Here's how the part is built. I have some questions about the finished solid (model axes, mm). A direction names the side the tool comes from. Coordinates: 2 decimals unless noted, no trailing zeros. Write each loop counter-clockwise with the first axis right and the second up, starting at its lowest first coordinate (ties: lowest second). Pieces come first, ordered by that corner, then holes. Notation, with made-up numbers: (-34.75, 52) -> (-27.75, 52) arc R12 ccw to (-27.75, 68) -> close; hole circle Ø9 at (5.5, 1). An arc over 180 degrees is marked (long way). Put each result on its own line as item: value.
```python
from build123d import *

# Parameters (mm, degrees)
SKETCH_1_W               = 42
SKETCH_1_H               = 42
EXTRUDE_1_DEPTH          = 65
SKETCH_2_R               = 18
EXTRUDE_2_DEPTH          = 22
EXTRUDE_3_DEPTH          = 19
SKETCH_4_R               = 11
EXTRUDE_4_DEPTH          = 2
SKETCH_6_W               = 43
SKETCH_6_H               = 1
CUT_EXTRUDE_1_DEPTH      = 2
PATTERN_CIRCULAR_1_COUNT = 4
HOLE_WIZARD_M3_1_D       = 2.5
HOLE_WIZARD_M3_1_DEPTH   = 7.5
HOLE_WIZARD_M3_1_TIP     = 0.751075774
SKETCH_9_W               = 16
SKETCH_9_H               = 9.5
EXTRUDE_5_DEPTH          = 8


with BuildPart() as part:
    # 草图1 → 凸台-拉伸1 (new body)
    with BuildSketch(Plane.XY):
        Rectangle(SKETCH_1_W, SKETCH_1_H)
    extrude(amount=EXTRUDE_1_DEPTH)

    # 草图2 → 凸台-拉伸2 (add)
    with BuildSketch(Plane.XY.offset(65)):
        Circle(SKETCH_2_R)
    extrude(amount=EXTRUDE_2_DEPTH)

    # 草图3 → 凸台-拉伸3 (add)
    with BuildSketch(Plane.XY.offset(87)):
        with BuildLine():
            Line((-2.645751311, 3), (2.645751311, 3))
            ThreePointArc((2.645751311, 3), (0, -4), (-2.645751311, 3))
        make_face()
    extrude(amount=EXTRUDE_3_DEPTH)

    # 草图4 → 凸台-拉伸4 (add)
    with BuildSketch(Plane.XY.offset(87)):
        Circle(SKETCH_4_R)
    extrude(amount=EXTRUDE_4_DEPTH)

    # 草图6 → 切除-拉伸1 (cut)
    with BuildSketch(Plane(origin=(0, 21, 0), x_dir=(1, 0, 0), z_dir=(0, 1, 0))):
        with Locations((0, -60)):
            Rectangle(SKETCH_6_W, SKETCH_6_H)
    cut_extrude_1 = extrude(amount=-CUT_EXTRUDE_1_DEPTH, mode=Mode.SUBTRACT)

    # 阵列(圆周)1: 切除-拉伸1 ×4 about axis
    pattern_circular_1_axis = Axis((0, 0, 0), (0, 0, 1))
    for i in range(1, PATTERN_CIRCULAR_1_COUNT):
        add(cut_extrude_1.rotate(pattern_circular_1_axis, i * 360 / PATTERN_CIRCULAR_1_COUNT), mode=Mode.SUBTRACT)

    # M3 螺纹孔1
    with Locations(Plane(origin=(-9.899494937, 9.899494937, 87), x_dir=(1, 0, 0), z_dir=(0, 0, 1))):
        with Locations((0, 0), (0, -19.798989874), (19.798989874, 0), (19.798989874, -19.798989874)):
            Hole(HOLE_WIZARD_M3_1_D / 2, depth=HOLE_WIZARD_M3_1_DEPTH)
            with Locations((0, 0, -(HOLE_WIZARD_M3_1_DEPTH + HOLE_WIZARD_M3_1_TIP / 2))):  # 118° drill point
                Cone(0, HOLE_WIZARD_M3_1_D / 2, HOLE_WIZARD_M3_1_TIP, mode=Mode.SUBTRACT)

    # 草图9 → 凸台-拉伸5 (add)
    with BuildSketch(Plane(origin=(0, 21, 0), x_dir=(1, 0, 0), z_dir=(0, 1, 0))):
        with Locations((0, -4.75)):
            Rectangle(SKETCH_9_W, SKETCH_9_H)
    extrude(amount=EXTRUDE_5_DEPTH)


solid = part.part
```
Item 1: If we mould it in two halves opening along Z, with no side actions, what happens to faces 5 (the flat face through (20, -2, 59.5)), 6 (the flat face through (0, -21, 29)), 7 (the flat face through (0, -1, 0)), 8 (the flat face through (20, -2, 60.5))? For each: released by +Z, released by -Z, zero draft, split by the parting line, or undercut.
Output:
face 5: undercut
face 6: zero draft
face 7: released by -Z
face 8: undercut
Item 2: Imagine slicing it at A-A on y = 0. Write out the boundary of the cut face in (x, z).
Output:
outline: (-21, 0) -> (21, 0) -> (21, 59.5) -> (19, 59.5) -> (19, 60.5) -> (21, 60.5) -> (21, 65) -> (18, 65) -> (18, 87) -> (11, 87) -> (11, 89) -> (4, 89) -> (4, 106) -> (-4, 106) -> (-4, 89) -> (-11, 89) -> (-11, 87) -> (-18, 87) -> (-18, 65) -> (-21, 65) -> (-21, 60.5) -> (-19, 60.5) -> (-19, 59.5) -> (-21, 59.5) -> close
Item 3: Imagine slicing it at D-D on y = -6.5. Write out the boundary of the cut face in (x, z), then the cut area to 3 significant figures.
Output:
outline: (-21, 0) -> (21, 0) -> (21, 59.5) -> (19, 59.5) -> (19, 60.5) -> (21, 60.5) -> (21, 65) -> (16.79, 65) -> (16.79, 87) -> (8.87, 87) -> (8.87, 89) -> (-8.87, 89) -> (-8.87, 87) -> (-16.79, 87) -> (-16.79, 65) -> (-21, 65) -> (-21, 60.5) -> (-19, 60.5) -> (-19, 59.5) -> (-21, 59.5) -> close
area: 3,500 mm²
Item 4: Imagine slicing it at C-C on z = 90.5. Write out the boundary of the cut face in (x, y), then the cut area to 3 significant figures.
Output:
outline: (-2.65, 3) arc R4 ccw (long way) to (2.65, 3) -> close
area: 46.6 mm²
Item 5: Please list where these lines run through material, in increasing order: line 1 along Y through (x, z) = (19, 38); line 2 along Z through (x, y) = (-4, -8); line 3 along Z through (x, y) = (-12, 4). Write a range as from..to.
Output:
line 1: y = -21..21
line 2: z = 0..89
line 3: z = 0..87
Item 6: Imagine slicing it at B-B on x = 0. Write out the boundary of the cut face in (y, z), then the cut area to 3 significant figures.
Output:
outline: (-21, 0) -> (29, 0) -> (29, 9.5) -> (21, 9.5) -> (21, 59.5) -> (19, 59.5) -> (19, 60.5) -> (21, 60.5) -> (21, 65) -> (18, 65) -> (18, 87) -> (11, 87) -> (11, 89) -> (3, 89) -> (3, 106) -> (-4, 106) -> (-4, 89) -> (-11, 89) -> (-11, 87) -> (-18, 87) -> (-18, 65) -> (-21, 65) -> (-21, 60.5) -> (-19, 60.5) -> (-19, 59.5) -> (-21, 59.5) -> close
area: 3,760 mm²
Item 7: For P1, Ø12, axis at x = -12, z = 80, coming from the -Y side; P2, Ø8, axis at x = 10, z = 17.5, coming from the +Y side; P3, Ø2, axis at x = -9.9, y = 9.9, coming from the +Z side, each with a flat end and sliding along its axis, tell me the tip position at first contact or that it passes through.
Output:
P1: stops at y = -16.97
P2: stops at y = 21
P3: stops at z = 79.35
Item 8: Which directions (+Z, -Z, +X, -X, +Y, -Y) give clear straight access to the entire face, cutting with the end or side of a thin tool? Please do faces 1 (the flat face through (0, 25, 9.5)), 2 (the cylindrical face through (10.17, -11.12, 83.2)), 3 (the flat face through (0, 29, 5)), 4 (the flat face through (8, 25, 5)).
Output:
face 1: +Z, +X, -X, +Y
face 2: +Z
face 3: +Z, -Z, +X, -X, +Y
face 4: +Z, -Z, +X, +Y
